Build history of the part. All positions in model axes, mm. A direction names the side the tool comes from. Round coordinates to 2 decimals unless told otherwise and drop trailing zeros. Write each loop counter-clockwise with the first axis right and the second up, starting at its lowest first coordinate (ties: lowest second). Pieces come first, ordered by that corner, then holes. Notation, with made-up numbers: M 63,29.25 L 71,29.25 A24 cw 71,58.25 Z; hole C -28,-25.5 d4. An arc over 180 degrees is marked long. Write item = value, one per line. Start each with the question number.
Q1. Band-saw the part on D-D on y = -2.1. State how many separate pieces and enclosed holes the cut face has, plus the area to 3 significant figures.
Q2. Band-saw the part on C-C on z = -10. Write the cut outline in (x, y).
Q3. Pull direction X, two halves, no side cores. Call faces 3 (the flat face through (-42.851, -2, -2)), 4 (the flat face through (-5, 0, -1)), 5 (the flat face through (51.015, -1.972, -20.119)), 6 (the flat face through (-31, -2, 3.451)): released by +X, released by -X, zero draft, split by the parting line, or undercut.
Q4. Band-saw the part on B-B on x = -8. Write the cut outline in (y, z).
Q5. Band-saw the part on A-A on x = 6. Write the cut outline in (y, z).
Q6. Drop a flat-ended pin along its axis: P1, Ø12.5, axis at x = 28, z = -2.5, coming from the -Y side. Give the stop position or say it passes through.
Q7. Probe L1, parallel to Z at x = -5.5, y = -1.7; L2, parallel to X at y = -4.3, z = 6.5; L3, parallel to X at y = -0.95, z = -1. List the from-to ranges inside material, lowest first.
Q8. Tool access for faces 1 (the flat face through (57.556, -2, -2)), 2 (the flat face through (-22.816, -2, -15)): list every direction of +Z, -Z, +X, -X, +Y, -Y with a clear straight run to the whole face (end or side of a thin tool).
```python
from build123d import *

# Parameters (mm, degrees)
F0_W     = 100.4062
F0_H     = 50.070776
F0_W_2   = 92.786201
F0_H_2   = 42.450776
F1_DEPTH = 4.572
F3_DEPTH = 4
F5_DEPTH = 4


with BuildPart() as f1:
    # F0 (on Front) → F1 (new body)
    with BuildSketch(Plane.XZ):
        with Locations((7.352479, -1.548582)):
            Rectangle(F0_W, F0_H)
        with Locations((7.352479, -1.548582)):
            Rectangle(F0_W_2, F0_H_2, mode=Mode.SUBTRACT)
    extrude(amount=F1_DEPTH)

    # F2 (on Front) → F3 (join)
    with BuildSketch(Plane.XZ):
        Polygon((47.517822, -23.616505), (54.588892, -16.545439), (39.591647, -1.548194), (54.532303, 13.392463), (47.461235, 20.463531), (32.520579, 5.522874), (17.569123, 20.47433), (10.498055, 13.403262), (25.449511, -1.548194), (10.608977, -16.388728), (17.680045, -23.459796), (32.520579, -8.619261), align=None)
    extrude(amount=F3_DEPTH)

    # F4 (on Front) → F5 (join)
    with BuildSketch(Plane.XZ):
        Polygon((-39.815622, 3.45103), (-39.815622, -6.54897), (-22.815622, -6.54897), (-22.815622, -23.54897), (-12.815622, -23.54897), (-12.815622, -6.54897), (4.184378, -6.54897), (4.184378, 3.45103), (-12.815622, 3.45103), (-12.815622, 20.45103), (-22.815622, 20.45103), (-22.815622, 3.45103), align=None)
    extrude(amount=F5_DEPTH)


solid = f1.part
```
Conclusion:
q1.separate_pieces = 1
q1.enclosed_holes = 8
q1.area = 2,790 mm^2
q2.outline = M -42.85,-4.57 L -39.04,-4.57 L -39.04,0 L -42.85,0 Z; M -22.82,-4 L -12.82,-4 L -12.82,0 L -22.82,0 Z; M 17,-4 L 31.14,-4 L 31.14,0 L 17,0 Z; M 33.9,-4 L 48.04,-4 L 48.04,0 L 33.9,0 Z; M 53.75,-4.57 L 57.56,-4.57 L 57.56,0 L 53.75,0 Z
q3.face_3 = released by -X
q3.face_4 = zero draft
q3.face_5 = undercut
q3.face_6 = undercut
q4.outline = M -4.57,-26.58 L 0,-26.58 L 0,-22.77 L -4.57,-22.77 Z; M -4.57,19.68 L 0,19.68 L 0,23.49 L -4.57,23.49 Z; M -4,-6.55 L 0,-6.55 L 0,3.45 L -4,3.45 Z
q5.outline = M -4.57,-26.58 L 0,-26.58 L 0,-22.77 L -4.57,-22.77 Z; M -4.57,19.68 L 0,19.68 L 0,23.49 L -4.57,23.49 Z
q6.P1 = -4
q7.L1 = -26.58 to -22.77, -6.55 to 3.45, 19.68 to 23.49
q7.L2 = -42.85 to -39.04, 53.75 to 57.56
q7.L3 = -42.85 to 4.18, 24.9 to 40.14, 53.75 to 57.56
q8.face_1 = +Z, -Z, +X, +Y, -Y
q8.face_2 = +Y, -Y
